The listing builds one solid part. Answer for the finished solid, in the listing's coordinates (mm). Round coordinates to 2 decimals unless told otherwise and drop trailing zeros. Write each loop counter-clockwise with the first axis right and the second up, starting at its lowest first coordinate (ties: lowest second). Pieces come first, ordered by that corner, then holes.
(1) Find the intervals of material crossed by probe 1 along X at (y, z) = (0, 479.5); probe 2 along Y at (x, z) = (0, 490); probe 3 along X at (y, z) = (-22.5, 30), in increasing order.
(2) This flat-tipped pin is pushed along its axis until it touches: pin 1 Ø1.5 at (x, y) = (4.5, -12) entering from +Z. Where does it stop, or does it pass through?
(3) A cutting plane is placed at A-A, the plane z = 39. Give the vertices of the cut face in (x, y), and give its area (3 significant figures).
from build123d import *

# Parameters (mm, degrees)
F0_W           = 98.0767756701
F0_H           = 69.9729025364
F1_DEPTH       = 508
F2_R           = 12.7
F4_D           = 22
F4_DEPTH       = 50.8
F4_CSINK_D     = 42
F4_CSINK_ANGLE = 90
F4_TIP         = 6.6094668093


with BuildPart() as f1:
    # F0 (on Top) → F1 (new body)
    with BuildSketch(Plane.XY):
        Rectangle(F0_W, F0_H)
    extrude(amount=F1_DEPTH)

    # F2
    f2_edges = [f1.edges().sort_by_distance(p)[0] for p in [
        (49.038388, 34.986451, 254),
        (-49.038388, 34.986451, 254),
        (-49.038388, -34.986451, 254),
        (49.038388, -34.986451, 254),
    ]]
    fillet(f2_edges, radius=F2_R)

    # F4
    with Locations(Plane.XY.offset(508)):
        with Locations((0, 0)):
            CounterSinkHole(F4_D / 2, F4_CSINK_D / 2, depth=F4_DEPTH, counter_sink_angle=F4_CSINK_ANGLE)
            with Locations((0, 0, -(F4_DEPTH + F4_TIP / 2))):  # 118° drill point
                Cone(0, F4_D / 2, F4_TIP, mode=Mode.SUBTRACT)


solid = f1.part
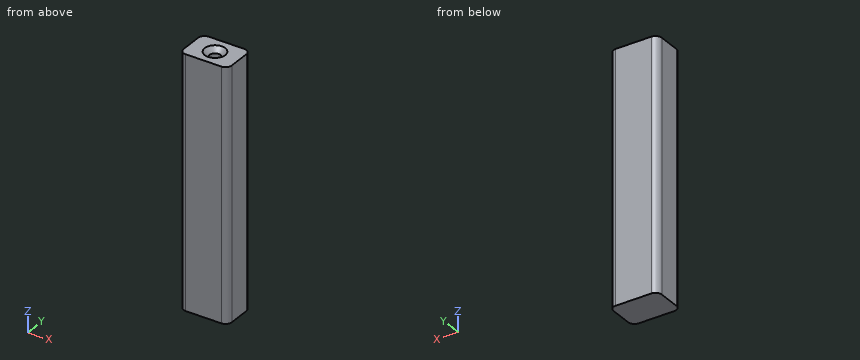
Solutions:
1. probe 1: x = -49.04 to -11, 11 to 49.04
1. probe 2: y = -34.99 to -11, 11 to 34.99
1. probe 3: x = -49.04 to 49.04
2. pin 1: stops at z = 500.57
3. outline: (-49.04, -22.29) arc R12.7 ccw to (-36.34, -34.99) - (36.34, -34.99) arc R12.7 ccw to (49.04, -22.29) - (49.04, 22.29) arc R12.7 ccw to (36.34, 34.99) - (-36.34, 34.99) arc R12.7 ccw to (-49.04, 22.29) - close
3. area: 6,720 mm2
